Could you check a few things on this model? Use its own coordinates, in mm. Face numbers are marked on the shaded views. A direction names the side the tool comes from. Round coordinates to 2 decimals unless told otherwise and drop trailing zeros. Loops run counter-clockwise (first coordinate to the right, second up) from the corner with the lowest first, then second, coordinate; pieces in that order, holes last. Notation, with made-up numbers: (10.25, -20.5) -> (67.25, -20.5) arc R25 cw to (67.25, 6.5) -> close; hole circle Ø1 at (57, -37). An arc over 180 degrees is marked (long way). Write each question's results on one line, items separated by ' | '.
from build123d import *

# Parameters (mm, degrees)
F1_DEPTH = 4
F2_DEPTH = 11
F3_R     = 2
F4_R     = 1


with BuildPart() as f1:
    # F0 (on Top) → F1 (new body)
    with BuildSketch(Plane.XY):
        Polygon((-12.696786, -0.35349), (-6.042262, -11.172484), (6.654524, -10.818994), (12.696786, 0.35349), (6.042262, 11.172484), (-6.654524, 10.818994), align=None)
        Polygon((-4.669021, -8.633283), (-9.811153, -0.273151), (-5.142132, 8.360132), (4.669021, 8.633283), (9.811153, 0.273151), (5.142132, -8.360132), align=None, mode=Mode.SUBTRACT)
        Polygon((-5.142132, 8.360132), (-9.811153, -0.273151), (-4.669021, -8.633283), (5.142132, -8.360132), (9.811153, 0.273151), (4.669021, 8.633283), align=None)
    extrude(amount=F1_DEPTH)

    # F0 (on Top) → F2 (join)
    with BuildSketch(Plane.XY):
        Polygon((-12.696786, -0.35349), (-6.042262, -11.172484), (6.654524, -10.818994), (12.696786, 0.35349), (6.042262, 11.172484), (-6.654524, 10.818994), align=None)
        Polygon((-4.669021, -8.633283), (-9.811153, -0.273151), (-5.142132, 8.360132), (4.669021, 8.633283), (9.811153, 0.273151), (5.142132, -8.360132), align=None, mode=Mode.SUBTRACT)
    extrude(amount=-F2_DEPTH)

    # F3
    f3_edges = [f1.edges().sort_by_distance(p)[0] for p in [
        (-0.306131, 10.995739, 4),
        (-9.675655, 5.232752, 4),
        (-9.369524, -5.762987, 4),
        (0.306131, -10.995739, 4),
        (9.675655, -5.232752, 4),
        (9.369524, 5.762987, 4),
    ]]
    fillet(f3_edges, radius=F3_R)

    # F4
    f4_edges = [f1.edges().sort_by_distance(p)[0] for p in [
        (-0.236556, 8.496708, -11),
        (-7.476643, 4.04349, -11),
        (-7.240087, -4.453217, -11),
        (0.236556, -8.496708, -11),
        (7.476643, -4.04349, -11),
        (7.240087, 4.453217, -11),
    ]]
    fillet(f4_edges, radius=F4_R)


solid = f1.part
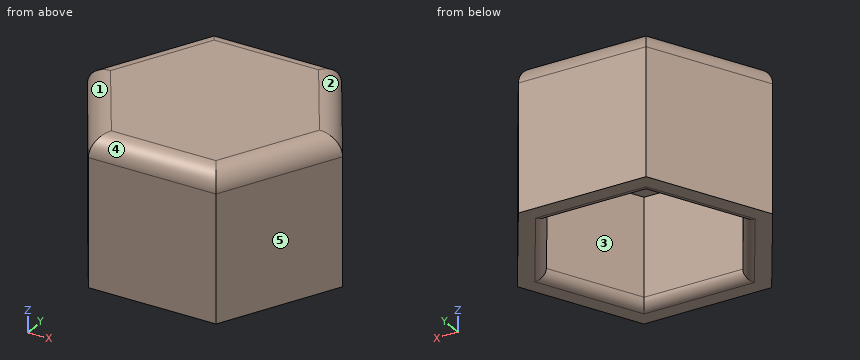
1) I want a section at C-C, the plane z = 1. Write out the boundary of the cut face in (x, y), plus the area to 3 significant figures.
Model answer:
outline: (-12.7, -0.35) -> (-6.04, -11.17) -> (6.65, -10.82) -> (12.7, 0.35) -> (6.04, 11.17) -> (-6.65, 10.82) -> close | area: 419 mm2
2) I need wall thicknesses on line 1 (Z direction, x = 6.5, y = 4.25); line 2 (Y direction, x = -4.5, z = -1.75); line 3 (Y direction, x = -0.75, z = -7.25). Which ranges of each line are inside material? Lowest first, please.
Model answer:
line 1: z = 0 to 4 | line 2: y = -11.13 to -8.63, 8.38 to 10.88 | line 3: y = -11.03 to -8.52, 8.48 to 10.98
3) For the marked faces 4 and 5, which set-ups out of +Z, -Z, +X, -X, +Y, -Y let a thin tool reach every point of the face, with its end or its side?
Model answer:
face 4: +Z, +X, -Y | face 5: +Z, -Z, +X, -Y
4) If we mould it in two halves opening along Y, with no side actions, what happens to the marked faces 1, 2 and 3? For each: released by +Y, released by -Y, zero draft, split by the parting line, or undercut.
Model answer:
face 1: released by -Y | face 2: released by +Y | face 3: undercut
5) I want a section at B-B, the plane z = 2.5. Write out the boundary of the cut face in (x, y), plus the area to 3 significant figures.
Model answer:
outline: (-12.62, -0.35) -> (-6.01, -11.11) -> (6.62, -10.76) -> (12.62, 0.35) -> (6.01, 11.11) -> (-6.62, 10.76) -> close | area: 414 mm2
6) I'm going to push flat-ended pins straight in: pin 1 (6 mm diameter, centred on y = 8, z = -2.5, fed in from -X); pin 2 (2 mm diameter, centred on x = -6.5, z = 0, fed in from +Y); pin 3 (6 mm diameter, centred on x = 9.5, z = -5.5, fed in from +Y). Where does each tip first touch, or does it pass through?
Model answer:
pin 1: stops at x = -9.8 | pin 2: stops at y = 10.85 | pin 3: stops at y = 10.43
7) I want a section at A-A, the plane z = -6.75. Write out the boundary of the cut face in (x, y).
Model answer:
outline: (-12.7, -0.35) -> (-6.04, -11.17) -> (6.65, -10.82) -> (12.7, 0.35) -> (6.04, 11.17) -> (-6.65, 10.82) -> close; hole (-9.81, -0.27) -> (-4.67, -8.63) -> (5.14, -8.36) -> (9.81, 0.27) -> (4.67, 8.63) -> (-5.14, 8.36) -> close
